from build123d import *

# Parameters (mm, degrees)
ESBO_O1_W                  = 125
ESBO_O1_H                  = 50
RESSALTO_EXTRUS_O1_DEPTH   = 2.5
ESBO_O2_R                  = 1.6
CORTE_EXTRUS_O2_DEPTH      = 2.5
CORTE_EXTRUS_O3_DEPTH      = 1.5
CORTE_EXTRUS_O5_DEPTH      = 113.726994752
CORTE_EXTRUS_O5_DEPTH_BACK = 113.726994752
ESBO_O12_R                 = 2.75
CORTE_EXTRUS_O6_DEPTH      = 2
ESBO_O19_R                 = 1.5
CORTE_EXTRUS_O7_DEPTH      = 2
FILETE1_R                  = 2


with BuildPart() as part:
    # Esboço1 → Ressalto-extrusão1 (new body)
    with BuildSketch(Plane.XY):
        with Locations((44.657564369, 9.905325444)):
            Rectangle(ESBO_O1_W, ESBO_O1_H)
    extrude(amount=RESSALTO_EXTRUS_O1_DEPTH)

    # Esboço2 → Corte-extrusão2 (cut)
    with BuildSketch(Plane.XY.offset(2.5)):
        with Locations((34.157564369, 22.905325444)):
            Circle(ESBO_O2_R)
        with Locations(Location((34.157564369, -3.094674556, 0), (0, 0, 180))):
            Circle(ESBO_O2_R)
        with Locations((52.157564369, -3.094674556)):
            Circle(ESBO_O2_R)
        with Locations(Location((52.157564369, 22.905325444, 0), (0, 0, 180))):
            Circle(ESBO_O2_R)
    extrude(amount=-CORTE_EXTRUS_O2_DEPTH, mode=Mode.SUBTRACT)

    # Esboço3 → Corte-extrusão3 (cut)
    with BuildSketch(Plane.XY.offset(2.5)):
        Polygon((-17.842435631, 32.905325444), (-17.842435631, 9.905325444), (-15.842435631, 9.905325444), (-15.842435631, 32.905325444), (107.157564369, 32.905325444), (107.157564369, 34.905325444), (-15.842435631, 34.905325444), (-17.842435631, 34.905325444), align=None)
        Polygon((-15.842435631, 9.905325444), (-17.842435631, 9.905325444), (-17.842435631, -13.094674556), (-17.842435631, -15.094674556), (-15.842435631, -15.094674556), (107.157564369, -15.094674556), (107.157564369, -13.094674556), (-15.842435631, -13.094674556), align=None)
    extrude(amount=-CORTE_EXTRUS_O3_DEPTH, mode=Mode.SUBTRACT)

    # Esboço4 → Corte-extrusão5 (cut, two sides: drawn at the far end of the back side and taken through both)
    with BuildSketch(Plane.XY.offset(2.5).offset(-CORTE_EXTRUS_O5_DEPTH_BACK)):
        Polygon((15.925055292, 9.905325444), (25.654023464, 29.905325444), (22.419553485, 29.905325444), (12.690585312, 9.905325444), (22.419553485, -10.094674556), (25.654023464, -10.094674556), align=None)
        Polygon((25.654023464, 23.738176067), (18.925055292, 9.905325444), (25.654023464, -3.927525179), align=None)
        Polygon((8.690585312, 9.905325444), (18.419553485, 29.905325444), (14.419553485, 29.905325444), (4.690585312, 9.905325444), (14.419553485, -10.094674556), (18.419553485, -10.094674556), align=None)
        Polygon((0.690585312, 9.905325444), (10.419553485, 29.905325444), (6.419553485, 29.905325444), (-3.309414688, 9.905325444), (6.419553485, -10.094674556), (10.419553485, -10.094674556), align=None)
        Polygon((-7.309414688, 9.905325444), (2.419553485, 29.905325444), (-1.580446515, 29.905325444), (-11.309414688, 9.905325444), (-1.580446515, -10.094674556), (2.419553485, -10.094674556), align=None)
        Polygon((85.895575254, -10.094674556), (95.624543426, 9.905325444), (85.895575254, 29.905325444), (81.895575254, 29.905325444), (91.624543426, 9.905325444), (81.895575254, -10.094674556), align=None)
        Polygon((77.895575254, -10.094674556), (87.624543426, 9.905325444), (77.895575254, 29.905325444), (73.895575254, 29.905325444), (83.624543426, 9.905325444), (73.895575254, -10.094674556), align=None)
        Polygon((69.895575254, -10.094674556), (79.624543426, 9.905325444), (69.895575254, 29.905325444), (65.895575254, 29.905325444), (75.624543426, 9.905325444), (65.895575254, -10.094674556), align=None)
        Polygon((71.624543426, 9.905325444), (61.895575254, 29.905325444), (58.661105274, 29.905325444), (68.390073446, 9.905325444), (58.661105274, -10.094674556), (61.895575254, -10.094674556), align=None)
        Polygon((65.390073446, 9.905325444), (58.661105274, -3.927525179), (58.661105274, 23.738176067), align=None)
    extrude(amount=CORTE_EXTRUS_O5_DEPTH + CORTE_EXTRUS_O5_DEPTH_BACK, mode=Mode.SUBTRACT)

    # Esboço12 → Corte-extrusão6 (cut)
    with BuildSketch(Plane.XY.offset(2.5)):
        with Locations((97.607564369, 24.905325444)):
            Circle(ESBO_O12_R)
        with Locations((97.607564369, -5.094674556)):
            Circle(ESBO_O12_R)
    extrude(amount=-CORTE_EXTRUS_O6_DEPTH, mode=Mode.SUBTRACT)

    # Esboço19 → Corte-extrusão7 (cut)
    with BuildSketch(Plane.XY.offset(0.5)):
        with Locations((97.607564369, 24.905325444)):
            Circle(ESBO_O19_R)
        with Locations((97.607564369, -5.094674556)):
            Circle(ESBO_O19_R)
    extrude(amount=-CORTE_EXTRUS_O7_DEPTH, mode=Mode.SUBTRACT)

    # Filete1
    filete1_edges = [part.edges().sort_by_distance(p)[0] for p in [
        (-17.842435631, -15.094674556, 0.5),
        (-15.842435631, -13.094674556, 1.75),
        (-17.842435631, 34.905325444, 0.5),
        (-15.842435631, 32.905325444, 1.75),
        (107.157564369, -15.094674556, 0.5),
        (107.157564369, -13.094674556, 1.75),
        (107.157564369, 32.905325444, 1.75),
        (107.157564369, 34.905325444, 0.5),
    ]]
    fillet(filete1_edges, radius=FILETE1_R - 0.0001)  # a hair under: the kernel refuses the full size


solid = part.part
Design review of the part built by this model. Coordinates are the model's own, in mm. Give positions to 0.01 mm unless a question says otherwise; leave off trailing zeros. Order: outer loops, then holes, each group sorted by start corner. A loop starts at its lowest first (then second) coordinate and runs counter-clockwise, first axis right, second up. Notation, with made-up numbers: (-37.75, 37.5) - (-4.75, 37.5) arc R33 cw to (-4.75, 66.5) - close; hole circle Ø2 at (26.25, 83). An arc over 180 degrees is marked (long way). Use CSV: the item, a comma, the result in double quotes. Start each with the question number.
Q1. Draft analysis for pull direction X (two halves, no side actions). For faces 1 (the face through (44, -14, 1)), 2 (the face through (25.654, 10, 1)), 3 (the face through (66.828, 19.765, 1.233)), state which applies: pulls with the +X half, pulls with the -X half, needs draft (parallel to the pull), parting line crosses it, or undercut.
Q2. Take a section at A-A (x = 89). State the section outline as (y, z) points.
Q3. Take a section at B-B (y = 14.5). Count the separate pieces of the cut face and the enclosed holes in it, and give its area (3 significant figures).
Q4. For line 1 (Y direction, x = -4.5, z = 0.3); line 2 (Y direction, x = 66.5, z = 1.8); line 3 (Y direction, x = -1, z = 1.9), list the stretches that pass through material, from the lowest coordinate up.
Q5. For P1, Ø1.5, axis at x = 64.5, z = 2, coming from the -Y side; P2, Ø0.8, axis at x = 72.5, z = 1.5, coming from the +Y side; P3, Ø1.2, axis at y = 8, z = 1.5, coming from the -X side, all flat-tipped, find the tip position at first contact; note any pin that passes through.
Calculated:
1,face 1,"needs draft"
1,face 2,"undercut"
1,face 3,"undercut"
2,outline,"(-15.09, 0) - (-3.71, 0) - (-3.71, 2.5) - (-13.09, 2.5) - (-13.09, 1) - (-15.09, 1) - close; (4.51, 0) - (15.3, 0) - (15.3, 2.5) - (4.51, 2.5) - close; (23.52, 0) - (34.91, 0) - (34.91, 1) - (32.91, 1) - (32.91, 2.5) - (23.52, 2.5) - close"
3,separate pieces,"11"
3,enclosed holes,"0"
3,area,"211 mm²"
4,line 1,"y = -15.09 to -4.09, 4.13 to 15.68, 23.9 to 34.91"
4,line 2,"y = -13.09 to -10.09, -8.85 to -0.63, 6.02 to 13.79, 20.44 to 28.66, 29.91 to 32.91"
4,line 3,"y = -13.09 to -10.09, -3.07 to 5.16, 14.65 to 22.88, 29.91 to 32.91"
5,P1,"stops at y = -13.09"
5,P2,"stops at y = 32.91"
5,P3,"stops at x = -17.84"
